```python
from build123d import *

# Parameters (mm, degrees)
SKETCH2_R           = 7.874
BOSS_EXTRUDE1_DEPTH = 586.74
BOSS_EXTRUDE3_DEPTH = 2.794
SKETCH4_R           = 9.144
BOSS_EXTRUDE4_DEPTH = 13.716
SKETCH6_R           = 4.7625
CUT_EXTRUDE1_DEPTH  = 0.254


with BuildPart() as part:
    # Sketch2 → Boss-Extrude1 (new body)
    with BuildSketch(Plane(origin=(0, 0, 0), x_dir=(1, 0, 0), z_dir=(0, 1, 0))):
        with Locations(Location((0, 0, 0), (0, 0, 270))):
            Circle(SKETCH2_R)
    extrude(amount=BOSS_EXTRUDE1_DEPTH)

    # Sketch3 → Boss-Extrude3 (add)
    with BuildSketch(Plane(origin=(0, 586.74, 0), x_dir=(1, 0, 0), z_dir=(0, 1, 0))):
        with BuildLine():
            ThreePointArc((-8.856145882, 6.172576861), (-9.973279553, 4.131067652), (-10.626911765, 1.897569853))
            ThreePointArc((-10.626911765, 1.897569853), (-12.7, 0), (-10.626911765, -1.897569853))
            ThreePointArc((-10.626911765, -1.897569853), (-9.973279553, -4.131067652), (-8.856145882, -6.172576861))
            ThreePointArc((-8.856145882, -6.172576861), (-8.980256121, -8.980256121), (-6.172576861, -8.856145882))
            ThreePointArc((-6.172576861, -8.856145882), (-4.131067652, -9.973279553), (-1.897569853, -10.626911765))
            ThreePointArc((-1.897569853, -10.626911765), (0, -12.7), (1.897569853, -10.626911765))
            ThreePointArc((1.897569853, -10.626911765), (4.131067652, -9.973279553), (6.172576861, -8.856145882))
            ThreePointArc((6.172576861, -8.856145882), (8.980256121, -8.980256121), (8.856145882, -6.172576861))
            ThreePointArc((8.856145882, -6.172576861), (9.973279553, -4.131067652), (10.626911765, -1.897569853))
            ThreePointArc((10.626911765, -1.897569853), (12.7, 0), (10.626911765, 1.897569853))
            ThreePointArc((10.626911765, 1.897569853), (9.973279553, 4.131067652), (8.856145882, 6.172576861))
            ThreePointArc((8.856145882, 6.172576861), (8.980256121, 8.980256121), (6.172576861, 8.856145882))
            ThreePointArc((6.172576861, 8.856145882), (4.131067652, 9.973279553), (1.897569853, 10.626911765))
            ThreePointArc((1.897569853, 10.626911765), (0, 12.7), (-1.897569853, 10.626911765))
            ThreePointArc((-1.897569853, 10.626911765), (-4.131067652, 9.973279553), (-6.172576861, 8.856145882))
            ThreePointArc((-6.172576861, 8.856145882), (-8.980256121, 8.980256121), (-8.856145882, 6.172576861))
        make_face()
    extrude(amount=BOSS_EXTRUDE3_DEPTH)

    # Sketch4 → Boss-Extrude4 (add)
    with BuildSketch(Plane(origin=(0, 589.534, 0), x_dir=(1, 0, 0), z_dir=(0, 1, 0))):
        with Locations(Location((0, 0, 0), (0, 0, 270))):
            Circle(SKETCH4_R)
    extrude(amount=BOSS_EXTRUDE4_DEPTH)

    # Sketch6 → Cut-Extrude1 (cut)
    with BuildSketch(Plane(origin=(0, 603.25, 0), x_dir=(1, 0, 0), z_dir=(0, 1, 0))):
        with Locations(Location((0, 0, 0), (0, 0, 270))):
            Circle(SKETCH6_R)
    extrude(amount=-CUT_EXTRUDE1_DEPTH, mode=Mode.SUBTRACT)


solid = part.part
```
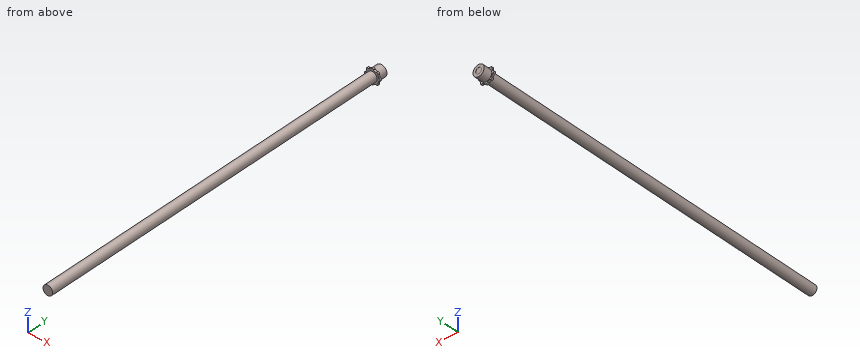
Check sheet for the modelled part. Datum: model origin and axes. Units: mm. Give positions to 0.01 mm unless a question says otherwise; leave off trailing zeros. Order: outer loops, then holes, each group sorted by start corner. A loop starts at its lowest first (then second) coordinate and runs counter-clockwise, first axis right, second up. Notation, with made-up numbers: M 87,51 L 132,51 A35 cw 132,90 Z; hole C -34,38.5 d8. An arc over 180 degrees is marked long. Answer in a Markdown table with one row per item.
1) Thickness scan on L1, parallel to X at y = 603.2, z = 0; L2, parallel to Y at x = 3.5, z = -2; L3, parallel to Y at x = 5.75, z = 7.5. Record the ranges inside material, lowest first. Write a range as [from, to].
Filled sheet:
| item | result |
|---|---|
| L1 | x = [-9.14, -4.76], [4.76, 9.14] |
| L2 | y = [0, 603] |
| L3 | y = [586.74, 589.53] |
2) Gauge pin test, flat ends, axial feed: P1, Ø10, axis at y = 205.5, z = -5.5, coming from the -X side; P2, Ø10, axis at y = 355.5, z = -7, coming from the +X side; P3, Ø8, axis at x = 7.5, y = 396.5, coming from the +Z side. Record the tip position at first contact, or that the pin passes through.
Filled sheet:
| item | result |
|---|---|
| P1 | stops at x = -7.86 |
| P2 | stops at x = 7.62 |
| P3 | stops at z = 7.05 |
3) Cross-section at A-A, the plane y = 230. Enter the section's corners in (x, z).
Filled sheet:
| item | result |
|---|---|
| outline | C 0,0 d15.75 |
